from build123d import *

# Parameters (mm, degrees)
F0_W     = 90
F0_H     = 90
F0_W_2   = 82.5
F0_H_2   = 82.5
F1_DEPTH = 700
F3_DEPTH = 90
F4_W     = 82.5
F4_H     = 82.5
F5_DEPTH = 40
F6_R     = 5.5
F7_DEPTH = 90.001


with BuildPart() as f1:
    # F0 (on Front) → F1 (new body)
    with BuildSketch(Plane.XZ):
        with Locations((45, 45)):
            Rectangle(F0_W, F0_H)
        with Locations((44.85, 44.85)):
            Rectangle(F0_W_2, F0_H_2, mode=Mode.SUBTRACT)
    extrude(amount=F1_DEPTH)

    # F2 (on face) → F3 (join)
    with BuildSketch(Plane.XY.offset(90)):
        Polygon((90, -700), (0, -700), (90, -732.757321), align=None)
    extrude(amount=-F3_DEPTH)

    # F4 (on face) → F5 (cut)
    with BuildSketch(Plane(origin=(0, -700, 0), x_dir=(-1, 0, 0), z_dir=(0, 1, 0))):
        with Locations((-44.85, 44.85)):
            Rectangle(F4_W, F4_H)
    extrude(amount=-F5_DEPTH, mode=Mode.SUBTRACT)

    # F6 (on face) → F7 (cut, through all)
    with BuildSketch(Plane.XY.offset(90)):
        with Locations((45, -30)):
            Circle(F6_R)
        with Locations((45, -60)):
            Circle(F6_R)
        with Locations((45, -90)):
            Circle(F6_R)
        with Locations((45, -120)):
            Circle(F6_R)
        with Locations((45, -150)):
            Circle(F6_R)
        with Locations((45, -180)):
            Circle(F6_R)
        with Locations((45, -210)):
            Circle(F6_R)
        with Locations((45, -240)):
            Circle(F6_R)
        with Locations((45, -270)):
            Circle(F6_R)
        with Locations((45, -300)):
            Circle(F6_R)
        with Locations((45, -330)):
            Circle(F6_R)
        with Locations((45, -360)):
            Circle(F6_R)
        with Locations((45, -390)):
            Circle(F6_R)
        with Locations((45, -420)):
            Circle(F6_R)
        with Locations((45, -450)):
            Circle(F6_R)
    extrude(amount=-F7_DEPTH, mode=Mode.SUBTRACT)


solid = f1.part
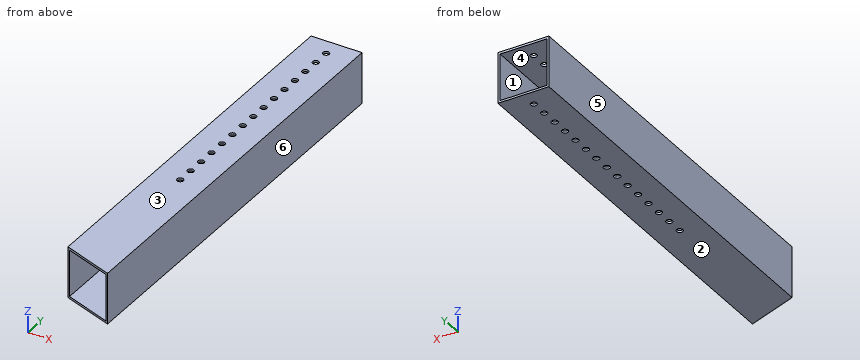
Design review of the part built by this model. Coordinates are the model's own, in mm. Face numbers are marked on the shaded views. A direction names the side the tool comes from. Coordinates: 2 decimals unless noted, no trailing zeros. Order: outer loops, then holes, each group sorted by start corner. A loop starts at its lowest first (then second) coordinate and runs counter-clockwise, first axis right, second up.
Item 1: For line 1 (Z direction, x = 45.5, y = -316); line 2 (X direction, y = -360, z = 1.4), list the stretches that pass through material, from the lowest coordinate up.
Item 2: Take a section at C-C, the plane y = -542. Write out the cut boundary in (x, z).
Item 3: For the marked faces 1 and 2, list the 3-axis set-ups (+Z, -Z, +X, -X, +Y, -Y) from which the entire face can be reached by the end or side of a thin tool; tool diameter is ignored.
Item 4: Take a section at A-A, the plane z = 70. Write out the cut boundary in (x, y).
Item 5: Take a section at B-B, the plane x = 21. Write out the cut boundary in (y, z).
Item 6: The part is to be moulded in two halves that separate along X. For the marked faces 3, 4, 5 and 6, say which applies: pulls with the +X half, pulls with the -X half, needs draft (parallel to the pull), parting line crosses it, or undercut.
Item 7: For pin 1 Ø14.5 at (x, y) = (45, -390) entering from +Z, flat-tipped, find the tip position at first contact; note if it passes through.
The answers:
1. line 1: z = 0 to 3.6, 86.1 to 90
1. line 2: x = 0 to 39.5, 50.5 to 90
2. outline: (0, 0) - (90, 0) - (90, 90) - (0, 90) - close; hole (3.6, 3.6) - (86.1, 3.6) - (86.1, 86.1) - (3.6, 86.1) - close
3. face 1: +Y, -Y
3. face 2: -Z, +X, -X, +Y, -Y
4. outline: (0, -700) - (3.6, -701.31) - (3.6, 0) - (0, 0) - close; (86.1, -731.34) - (90, -732.76) - (90, 0) - (86.1, 0) - close
5. outline: (-707.64, 0) - (0, 0) - (0, 3.6) - (-707.64, 3.6) - close; (-707.64, 86.1) - (0, 86.1) - (0, 90) - (-707.64, 90) - close
6. face 3: needs draft
6. face 4: undercut
6. face 5: pulls with the -X half
6. face 6: pulls with the +X half
7. pin 1: stops at z = 90
